Study the drawing (mm; zero at the part's minimum x, y, z) and answer. A direction names the side the tool comes from. Round coordinates to 2 decimals unless told otherwise and drop trailing zeros. Loops run counter-clockwise (first coordinate to the right, second up) from the corner with the lowest first, then second, coordinate; pieces in that order, holes last. Notation, with made-up numbers: (46, -11) -> (81, -11) arc R19 cw to (81, 9) -> close; hole circle Ø4 at (1.5, 43.25). An arc over 180 degrees is marked (long way). Write each question's results on one line, items separated by ' | '. Start each with the question number.
(1) The part is cut by section B-B (z = 6.35). Determine the outline of the cut face in (x, y).
(2) Flat-ended cylindrical pins translate along their axes: pin 1 (7.5 mm diameter, centred on x = 6.35, z = 6.35, fed in from -Y); pin 2 (4 mm diameter, centred on x = 2, y = 8, fed in from +Z); pin 3 (3 mm diameter, centred on x = 8.5, y = 7, fed in from +Z); pin 4 (2 mm diameter, centred on y = 1.5, z = 6, fed in from -X). Find the tip coordinate at first contact, or state that the pin passes through.
(3) The part is cut by section D-D (z = 9.5). Determine the outline of the cut face in (x, y) (1 decimal).
(4) Determine the mould class of the marked faces 1, 2 and 3 for opening direction X: released by +X, released by -X, zero draft, split by the parting line, or undercut.
(5) For the marked faces 4 and 5, determine the directions among +Z, -Z, +X, -X, +Y, -Y from which every point of the face is accessible in a straight line to the end or side of a thin tool.
(6) The part is cut by section A-A (x = 6.35). Determine the outline of the cut face in (y, z).
(7) Straight lines are drawn through the part: probe 1 along Z at (x, y) = (6.35, 5.5); probe 2 along Z at (x, y) = (6.35, 4.5). For each, find the intervals that lie inside material, in ascending order.
(8) The part is cut by section C-C (y = 2.5). Determine the outline of the cut face in (x, z).
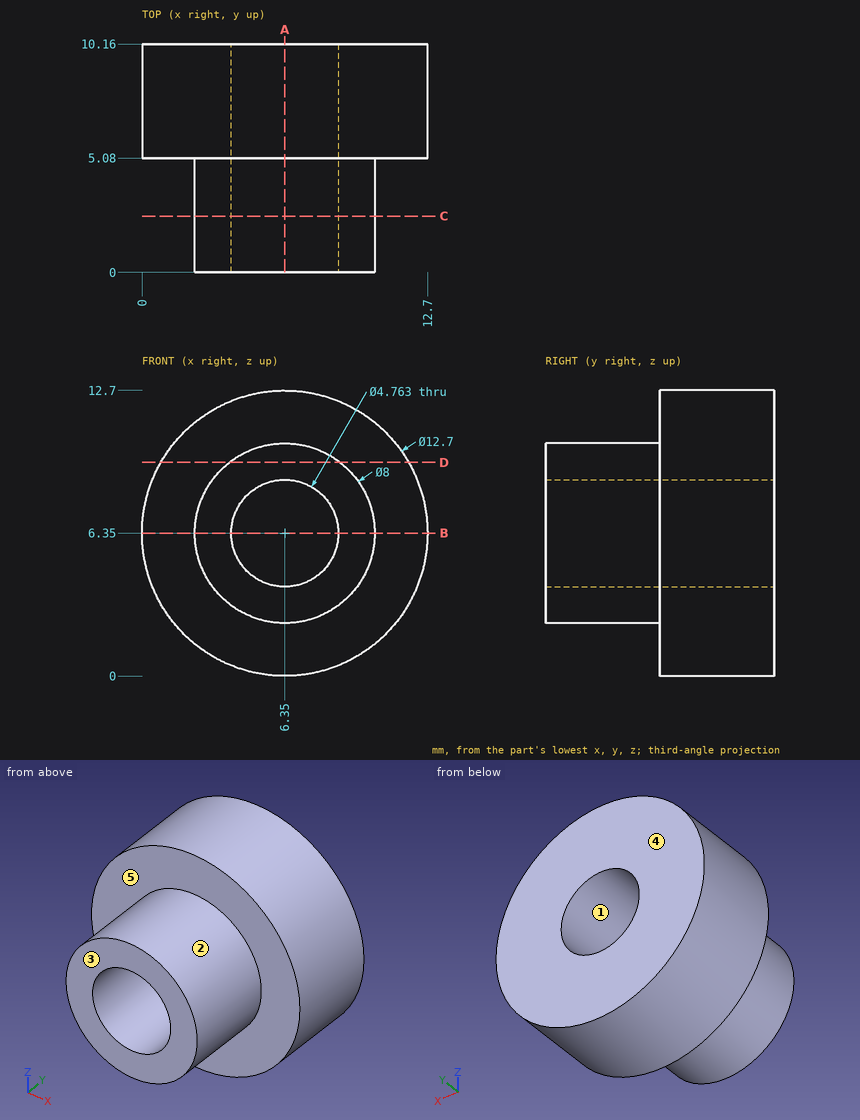
Checked values:
1) outline: (0, 5.08) -> (2.35, 5.08) -> (2.35, 0) -> (3.97, 0) -> (3.97, 10.16) -> (0, 10.16) -> close; (8.73, 0) -> (10.35, 0) -> (10.35, 5.08) -> (12.7, 5.08) -> (12.7, 10.16) -> (8.73, 10.16) -> close
2) pin 1: stops at y = 0 | pin 2: stops at z = 12.25 | pin 3: stops at z = 12.67 | pin 4: stops at x = 2.35
3) outline: (0.8, 5.1) -> (3.9, 5.1) -> (3.9, 0) -> (8.8, 0) -> (8.8, 5.1) -> (11.9, 5.1) -> (11.9, 10.2) -> (0.8, 10.2) -> close
4) face 1: undercut | face 2: split by the parting line | face 3: zero draft
5) face 4: +Z, -Z, +X, -X, +Y | face 5: -Y
6) outline: (0, 2.35) -> (5.08, 2.35) -> (5.08, 0) -> (10.16, 0) -> (10.16, 3.97) -> (0, 3.97) -> close; (0, 8.73) -> (10.16, 8.73) -> (10.16, 12.7) -> (5.08, 12.7) -> (5.08, 10.35) -> (0, 10.35) -> close
7) probe 1: z = 0 to 3.97, 8.73 to 12.7 | probe 2: z = 2.35 to 3.97, 8.73 to 10.35
8) outline: circle Ø8 at (6.35, 6.35); hole circle Ø4.76 at (6.35, 6.35)
